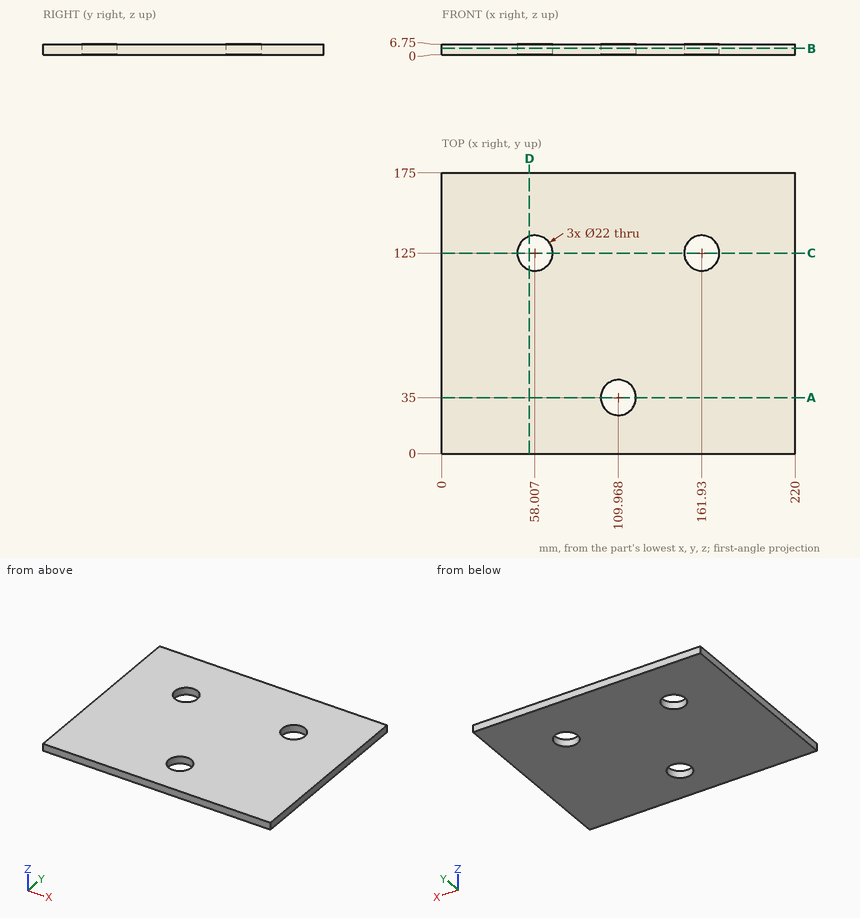
Input: dimensioned drawing with shaded views. Units: mm. Origin: part minimum x, y, z. Round coordinates to 2 decimals unless told otherwise and drop trailing zeros. Order: outer loops, then holes, each group sorted by start corner. A loop starts at its lowest first (then second) coordinate and runs counter-clockwise, first axis right, second up.
1. Cut plane C-C, the plane y = 125. Output: boundary loops of the cut face in (x, z), then the cut area to 3 significant figures.
The answers:
outline: (0, 0) - (47.01, 0) - (47.01, 6.75) - (0, 6.75) - close; (69.01, 0) - (150.93, 0) - (150.93, 6.75) - (69.01, 6.75) - close; (172.93, 0) - (220, 0) - (220, 6.75) - (172.93, 6.75) - close
area: 1,190 mm2
2. Cut plane A-A, the plane y = 35. Output: boundary loops of the cut face in (x, z), then the cut area to 3 significant figures.
The answers:
outline: (0, 0) - (98.97, 0) - (98.97, 6.75) - (0, 6.75) - close; (120.97, 0) - (220, 0) - (220, 6.75) - (120.97, 6.75) - close
area: 1,340 mm2
3. Cut plane D-D, the plane x = 54.5. Output: boundary loops of the cut face in (y, z).
The answers:
outline: (0, 0) - (114.57, 0) - (114.57, 6.75) - (0, 6.75) - close; (135.43, 0) - (175, 0) - (175, 6.75) - (135.43, 6.75) - close
4. Cut plane B-B, the plane z = 4. Output: boundary loops of the cut face in (x, y), then the cut area to 3 significant figures.
The answers:
outline: (0, 0) - (220, 0) - (220, 175) - (0, 175) - close; hole circle Ø22 at (58.01, 125); hole circle Ø22 at (109.97, 35); hole circle Ø22 at (161.93, 125)
area: 37,400 mm2
5. Material intervals for line 1 (Y direction, x = 162.5, z = 5.25) (1 decimal); line 2 (Y direction, x = 103, z = 2.75), sorted ascending.
The answers:
line 1: y = 0 to 114, 136 to 175
line 2: y = 0 to 26.49, 43.51 to 175
